```python
from build123d import *

# Parameters (mm, degrees)
BOSS_EXTRUDE1_DEPTH = 3.25
SKETCH2_W           = 0.5
SKETCH2_H           = 4
BOSS_EXTRUDE2_DEPTH = 2
SKETCH3_R           = 1.25
CUT_EXTRUDE1_DEPTH  = 14


with BuildPart() as part:
    # Sketch1 → Boss-Extrude1 (new, symmetric)
    with BuildSketch(Plane(origin=(0, 0, 0), x_dir=(1, 0, 0), z_dir=(0, 1, 0))):
        Polygon((0, 9.5), (9.5, 9.5), (10.5, 10.5), (20, 10.5), (20, 0), (0, 0), align=None)
    extrude(amount=BOSS_EXTRUDE1_DEPTH, both=True)

    # Sketch2 → Boss-Extrude2 (add, symmetric)
    with BuildSketch(Plane(origin=(0, 0, 0), x_dir=(1, 0, 0), z_dir=(0, 1, 0))):
        Polygon((17, 10.5), (17, 11.5), (-21.610231805, 17), (-21.680744625, 16.504997028), (16.5, 11.066177171), (16.5, 10.5), align=None)
        with Locations((18.25, -2)):
            Rectangle(SKETCH2_W, SKETCH2_H)
        with Locations((9.25, -2)):
            Rectangle(SKETCH2_W, SKETCH2_H)
        with Locations((1.75, -2)):
            Rectangle(SKETCH2_W, SKETCH2_H)
    extrude(amount=BOSS_EXTRUDE2_DEPTH, both=True)

    # Sketch3 → Cut-Extrude1 (cut)
    with BuildSketch(Plane(origin=(0, 3.25, 0), x_dir=(1, 0, 0), z_dir=(0, 1, 0))):
        with Locations(Location((5.25, 3.05, 0), (0, 0, 270))):
            Circle(SKETCH3_R)
        with Locations(Location((14.75, 3.05, 0), (0, 0, 270))):
            Circle(SKETCH3_R)
    extrude(amount=-CUT_EXTRUDE1_DEPTH, mode=Mode.SUBTRACT)


solid = part.part
```
Geometry: final body of the model. Coordinates: model frame, mm. A direction names the side the tool comes from. Round coordinates to 2 decimals unless told otherwise and drop trailing zeros. Loops run counter-clockwise (first coordinate to the right, second up) from the corner with the lowest first, then second, coordinate; pieces in that order, holes last.
Item 1: Line query: L1, parallel to X at y = -0.5, z = -3.05; L2, parallel to X at y = 1.5, z = 0.75; L3, parallel to Z at x = 5.5, y = -1.5. Output: solid intervals per line, ascending.
Checked values:
L1: x = 0 to 4, 6.5 to 13.5, 16 to 20
L2: x = 1.5 to 2, 9 to 9.5, 18 to 18.5
L3: z = -13.14 to -12.63, -9.5 to -4.27, -1.83 to 0
Item 2: Section C-C, the plane x = 12. Output: boundary loops of the cut face in (y, z).
Checked values:
outline: (-3.25, -10.5) - (3.25, -10.5) - (3.25, 0) - (-3.25, 0) - close; (-2, -12.21) - (2, -12.21) - (2, -11.71) - (-2, -11.71) - close
Item 3: Mould query, pull axis Z, two halves, no side actions, for faces 1 (the flat face through (2, 0, 2)), 2 (the flat face through (-2.03, -0.03, -14.21)), 3 (the flat face through (15, 0, -10.5)). Classes: released by +Z, released by -Z, zero draft, split by the parting line, or undercut.
Checked values:
face 1: zero draft
face 2: released by -Z
face 3: undercut
Item 4: Section B-B, the plane y = -0.75. Output: boundary loops of the cut face in (x, z) (3 decimals).
Checked values:
outline: (-21.681, -16.505) - (-21.61, -17) - (17, -11.5) - (17, -10.5) - (20, -10.5) - (20, 0) - (18.5, 0) - (18.5, 4) - (18, 4) - (18, 0) - (9.5, 0) - (9.5, 4) - (9, 4) - (9, 0) - (2, 0) - (2, 4) - (1.5, 4) - (1.5, 0) - (0, 0) - (0, -9.5) - (9.5, -9.5) - (10.5, -10.5) - (16.5, -10.5) - (16.5, -11.066) - close; hole circle Ø2.5 at (5.25, -3.05); hole circle Ø2.5 at (14.75, -3.05)
Item 5: Reachability of faces 4 (the flat face through (18.5, 0, 2)), 5 (the flat face through (5, 0, -9.5)), 6 (the flat face through (9.5, 0, 2)), 7 (the flat face through (-2, -2, -14)), 8 (the flat face through (17, 0, -11)) from +Z, -Z, +X, -X, +Y, -Y: full face, straight path, thin tool, end or side. Return the list, or none.
Checked values:
face 4: +Z, +X, +Y, -Y
face 5: -X, +Y, -Y
face 6: +Z, +Y, -Y
face 7: -Z, +X, -X, -Y
face 8: -Z, +X, +Y, -Y
Item 6: Section A-A, the plane z = -3.05. Output: boundary loops of the cut face in (x, y), plus the area to 3 significant figures.
Checked values:
outline: (0, -3.25) - (4, -3.25) - (4, 3.25) - (0, 3.25) - close; (6.5, -3.25) - (13.5, -3.25) - (13.5, 3.25) - (6.5, 3.25) - close; (16, -3.25) - (20, -3.25) - (20, 3.25) - (16, 3.25) - close
area: 97.5 mm2
Item 7: Contact query for flat-ended pins moving along their axis: P1, Ø0.6, axis at x = 9.5, z = 1.5, coming from the -Y side; P2, Ø1.2, axis at y = 1, z = 2, coming from the -X side; P3, Ø2, axis at x = -17, y = -2.5, coming from the +Z side. Output: stop coordinate, or through.
Checked values:
P1: stops at y = -2
P2: stops at x = 1.5
P3: stops at z = -15.71
Item 8: Section D-D, the plane x = 5.25. Output: boundary loops of the cut face in (y, z).
Checked values:
outline: (-3.25, -9.5) - (3.25, -9.5) - (3.25, -4.3) - (-3.25, -4.3) - close; (-3.25, -1.8) - (3.25, -1.8) - (3.25, 0) - (-3.25, 0) - close; (-2, -13.17) - (2, -13.17) - (2, -12.67) - (-2, -12.67) - close
